Could you check a few things on this drawing? It's one solid part, dimensions in mm from its lowest x, y, z. A direction names the side the tool comes from. Give positions to 0.01 mm unless a question says otherwise; leave off trailing zeros. Loops run counter-clockwise (first coordinate to the right, second up) from the corner with the lowest first, then second, coordinate; pieces in that order, holes last. Notation, with made-up numbers: (62, 10) - (83, 10) arc R32 ccw to (83, 47) - close; hole circle Ø4 at (9.25, 13.25). An arc over 180 degrees is marked (long way). Use a Markdown table: item, result.
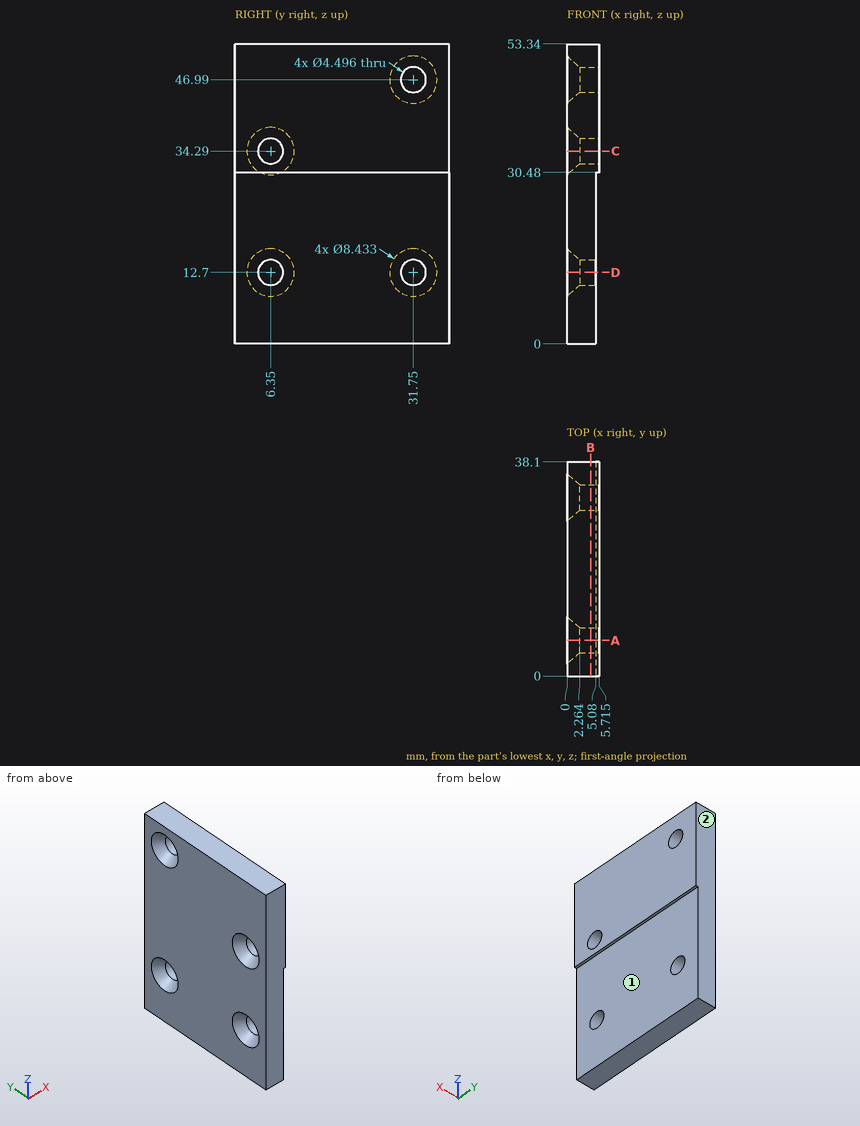
(1) On a 3-axis mill with a long thin cutter (end or side, diameter ignored), from which of +Z, -Z, +X, -X, +Y, -Y can I reach the whole of each face in a straight line? I mean the marked faces 1 and 2. Say none if no direction works.
A:
| item | result |
|---|---|
| face 1 | -Z, +X, +Y, -Y |
| face 2 | +Z, -Z, +X, -X, +Y |
(2) Suppose I cut it at D-D on z = 12.7. Write out the boundary of the cut face in (x, y) (1 decimal).
A:
| item | result |
|---|---|
| outline | (0, 0) - (5.1, 0) - (5.1, 4.1) - (2.3, 4.1) - (0, 2.1) - close; (0, 10.6) - (2.3, 8.6) - (5.1, 8.6) - (5.1, 29.5) - (2.3, 29.5) - (0, 27.5) - close; (0, 36) - (2.3, 34) - (5.1, 34) - (5.1, 38.1) - (0, 38.1) - close |
(3) If I drill on line 1 (Y direction, x = 4.45, z = 12.7); line 2 (Z direction, x = 3.35, y = 31.75); line 3 (Z direction, x = 4.6, y = 7), over which ranges is the centre line in solid material (lowest first)?
A:
| item | result |
|---|---|
| line 1 | 0 to 4.1, 8.6 to 29.5, 34 to 38.1 |
| line 2 | 0 to 10.45, 14.95 to 44.74, 49.24 to 53.34 |
| line 3 | 0 to 10.55, 14.85 to 32.14, 36.44 to 53.34 |
(4) Suppose I cut it at A-A on y = 6.35. Write out the boundary of the cut face in (x, z) (1 decimal), plus the area to 3 significant figures.
A:
| item | result |
|---|---|
| outline | (0, 0) - (5.1, 0) - (5.1, 10.5) - (2.3, 10.5) - (0, 8.5) - close; (0, 16.9) - (2.3, 14.9) - (5.1, 14.9) - (5.1, 30.5) - (5.7, 30.5) - (5.7, 32) - (2.3, 32) - (0, 30.1) - close; (0, 38.5) - (2.3, 36.5) - (5.7, 36.5) - (5.7, 53.3) - (0, 53.3) - close |
| area | 228 mm2 |
(5) Suppose I cut it at C-C on z = 34.29. Write out the boundary of the cut face in (x, y) (1 decimal).
A:
| item | result |
|---|---|
| outline | (0, 0) - (5.7, 0) - (5.7, 4.1) - (2.3, 4.1) - (0, 2.1) - close; (0, 10.6) - (2.3, 8.6) - (5.7, 8.6) - (5.7, 38.1) - (0, 38.1) - close |
(6) Will these pins go through, and if not, where does the flat tip stop? pin 1 (0.7 mm diameter, centred on x = 5.5, y = 26.5, fed in from -Z); pin 2 (1.5 mm diameter, centred on x = 2, z = 36.5, fed in from -Y); pin 3 (2 mm diameter, centred on y = 9.5, z = 12.5, fed in from -X); pin 4 (15 mm diameter, centred on y = 17, z = 10, fed in from +X).
A:
| item | result |
|---|---|
| pin 1 | z = 30.48 |
| pin 2 | y = 0 |
| pin 3 | x = 0.07 |
| pin 4 | x = 5.08 |
(7) Suppose I cut it at B-B on x = 4.2. Count the separate pieces of the cut face and the enclosed holes in it, plus the area to 3 significant figures.
A:
| item | result |
|---|---|
| separate pieces | 1 |
| enclosed holes | 4 |
| area | 1,970 mm2 |
